```python
from build123d import *

# Parameters (mm, degrees)
SKETCH1_W           = 115
SKETCH1_H           = 115
BOSS_EXTRUDE1_DEPTH = 6.5
SKETCH2_W           = 89
SKETCH2_H           = 89
BOSS_EXTRUDE2_DEPTH = 806.45
FILLET1_R           = 7.5
SKETCH3_R           = 3.3782
CUT_EXTRUDE1_DEPTH  = 6.5
SHELL1_T            = -5


with BuildPart() as part:
    # Sketch1 → Boss-Extrude1 (new body)
    with BuildSketch(Plane.XY):
        Rectangle(SKETCH1_W, SKETCH1_H)
    extrude(amount=BOSS_EXTRUDE1_DEPTH)

    # Sketch2 → Boss-Extrude2 (add)
    with BuildSketch(Plane.XY.offset(6.5)):
        Rectangle(SKETCH2_W, SKETCH2_H)
    extrude(amount=BOSS_EXTRUDE2_DEPTH)

    # Fillet1
    fillet1_edges = [part.edges().sort_by_distance(p)[0] for p in [
        (44.5, -44.5, 409.725),
        (44.5, 44.5, 409.725),
        (-44.5, 44.5, 409.725),
        (-44.5, -44.5, 409.725),
        (57.5, -57.5, 3.25),
        (-57.5, -57.5, 3.25),
        (-57.5, 57.5, 3.25),
        (57.5, 57.5, 3.25),
    ]]
    fillet(fillet1_edges, radius=FILLET1_R)

    # Sketch3 → Cut-Extrude1 (cut)
    with BuildSketch(Plane.XY.offset(6.5)):
        with Locations((48, -48)):
            Circle(SKETCH3_R)
        with Locations((-48, 48)):
            Circle(SKETCH3_R)
        with Locations((48, 48)):
            Circle(SKETCH3_R)
        with Locations((-48, -48)):
            Circle(SKETCH3_R)
    extrude(amount=-CUT_EXTRUDE1_DEPTH, mode=Mode.SUBTRACT)

    # Shell1
    shell1_openings = [part.faces().sort_by_distance(p)[0] for p in [
        (-51.3782, -48, 0),
    ]]
    offset(amount=SHELL1_T, openings=shell1_openings, kind=Kind.INTERSECTION)


solid = part.part
```
Could you check a few things on this model? Use its own coordinates, in mm. A direction names the side the tool comes from. Round coordinates to 2 decimals unless told otherwise and drop trailing zeros. Loops run counter-clockwise (first coordinate to the right, second up) from the corner with the lowest first, then second, coordinate; pieces in that order, holes last. Notation, with made-up numbers: (60.25, -29) - (87.25, -29) arc R30 cw to (87.25, -5) - close; hole circle Ø8 at (61, -6.5). An arc over 180 degrees is marked (long way). Use CSV: the item, a comma, the result in double quotes.
Item 1: If we section it at A-A on z = 671.5: List the corners of the cut face in (x, y) for me, then the cut area to 3 significant figures.
Here are the results:
outline,"(-44.5, -37) arc R7.5 ccw to (-37, -44.5) - (37, -44.5) arc R7.5 ccw to (44.5, -37) - (44.5, 37) arc R7.5 ccw to (37, 44.5) - (-37, 44.5) arc R7.5 ccw to (-44.5, 37) - close; hole (-39.5, -37) arc R2.5 ccw to (-37, -39.5) - (37, -39.5) arc R2.5 ccw to (39.5, -37) - (39.5, 37) arc R2.5 ccw to (37, 39.5) - (-37, 39.5) arc R2.5 ccw to (-39.5, 37) - close"
area,"1,640 mm²"
Item 2: If we mould it in two halves opening along Y, with no side actions, what happens to faces 1 (the flat face through (0, -55, 0)), 2 (the flat face through (-1, 39.5, 399)), 3 (the flat face through (-1, -44.5, 404))? For each: pulls with the +Y half, pulls with the -Y half, needs draft (parallel to the pull), parting line crosses it, or undercut.
Here are the results:
face 1,"needs draft"
face 2,"undercut"
face 3,"pulls with the -Y half"
Item 3: For faces 4 (the flat face through (-52, 1, 6.5)), 5 (the flat face through (44.5, -1, 404)), 6 (the flat face through (-1, -39.5, 399)), which set-ups out of +Z, -Z, +X, -X, +Y, -Y let a thin tool reach every point of the face, with its end or its side?
Here are the results:
face 4,"+Z"
face 5,"+Z, +X, +Y, -Y"
face 6,"-Z"
Item 4: If we section it at B-B on y = 5.5: List the corners of the cut face in (x, z) for me.
Here are the results:
outline,"(-57.5, 0) - (-52.5, 0) - (-52.5, 1.5) - (-39.5, 1.5) - (-39.5, 807.95) - (39.5, 807.95) - (39.5, 1.5) - (52.5, 1.5) - (52.5, 0) - (57.5, 0) - (57.5, 6.5) - (44.5, 6.5) - (44.5, 812.95) - (-44.5, 812.95) - (-44.5, 6.5) - (-57.5, 6.5) - close"
Item 5: I need wall thicknesses on L1, parallel to Y at x = -48, z = 2; L2, parallel to X at y = -25.5, z = 344.5. Which ranges of each line are inside material? Lowest first, please. Write a range as [from, to].
Here are the results:
L1,"y = [-57.5, -51.38], [-44.62, 44.62], [51.38, 57.5]"
L2,"x = [-44.5, -39.5], [39.5, 44.5]"
Item 6: Will these pins go through, and if not, where does the flat tip stop? pin 1 (1 mm diameter, centred on x = 25, z = 324, fed in from -Y); pin 2 (22 mm diameter, centred on x = -4, z = 525.5, fed in from +Y); pin 3 (6 mm diameter, centred on x = -48, y = 48, fed in from -Z); pin 4 (1 mm diameter, centred on y = -32.5, z = 645, fed in from +X).
Here are the results:
pin 1,"stops at y = -44.5"
pin 2,"stops at y = 44.5"
pin 3,"passes through"
pin 4,"stops at x = 44.5"
